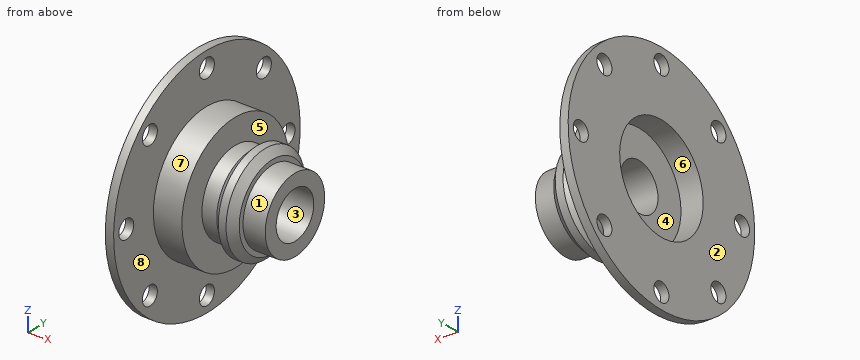
```python
from build123d import *

# Parameters (mm, degrees)
F2_R     = 4
F3_DEPTH = 3.551


with BuildPart() as f1:
    # F0 (on Front) → F1 (revolve)
    with BuildSketch(Plane.XZ):
        Polygon((-31.7, 10.0325), (0, 10.0325), (0, 15.85), (-9.5, 15.85), (-9.5, 17.875), (-12.625, 21), (-15.975, 21), (-19.1, 17.875), (-25.45, 17.875), (-25.45, 28.55), (-37.65, 28.55), (-37.65, 49.75), (-41.2, 49.75), (-41.2, 22.275), (-31.7, 22.275), align=None)
    revolve(axis=Axis((-20.6, 0, 0), (-1, 0, 0)))

    # F2 (on face) → F3 (cut, through all)
    with BuildSketch(Plane.YZ.offset(-37.65)):
        with Locations((0, 43)):
            Circle(F2_R)
        with Locations((30.405592, 30.405592)):
            Circle(F2_R)
        with Locations((43, 0)):
            Circle(F2_R)
        with Locations((30.405592, -30.405592)):
            Circle(F2_R)
        with Locations((0, -43)):
            Circle(F2_R)
        with Locations((-30.405592, -30.405592)):
            Circle(F2_R)
        with Locations((-43, 0)):
            Circle(F2_R)
        with Locations((-30.405592, 30.405592)):
            Circle(F2_R)
    extrude(amount=-F3_DEPTH, mode=Mode.SUBTRACT)


solid = f1.part
```
Geometry: final body of the model. Coordinates: model frame, mm. Face numbers are marked on the shaded views. A direction names the side the tool comes from. Coordinates: 2 decimals unless noted, no trailing zeros. Order: outer loops, then holes, each group sorted by start corner. A loop starts at its lowest first (then second) coordinate and runs counter-clockwise, first axis right, second up. Notation, with made-up numbers: (39.5, 40) -> (52.5, 40) arc R17 cw to (52.5, 55) -> close; hole circle Ø8 at (82.25, 64). An arc over 180 degrees is marked (long way). Answer in a Markdown table with one row per item.
Item 1: Contact query for flat-ended pins moving along their axis: P1, Ø9, axis at y = 0, z = -43, coming from the +X side; P2, Ø5, axis at x = -27, y = -3, coming from the +Z side; P3, Ø8, axis at x = -8.5, z = -9.5, coming from the +Y side. Output: stop coordinate, or through.
Return value:
| item | result |
|---|---|
| P1 | stops at x = -37.65 |
| P2 | stops at z = 28.55 |
| P3 | stops at y = 18.97 |
Item 2: Access query for the marked faces 1, 2, 3, 4 and 5. Directions: +Z, -Z, +X, -X, +Y, -Y. A direction counts if a zero-diameter tool reaches every point of the face in a straight line with its end or side. Return the directions, or none.
Return value:
| item | result |
|---|---|
| face 1 | +X |
| face 2 | +Z, -Z, -X, +Y, -Y |
| face 3 | +X, -X |
| face 4 | -X |
| face 5 | none |
Item 3: Ray query, L1, parallel to Y at x = -37.5, z = 0 (3 decimals); L2, parallel to X at y = 38, z = -17; L3, parallel to X at y = 10, z = -24.5. Return the intervals inside material, ascending.
Return value:
| item | result |
|---|---|
| L1 | y = -28.55 to -22.275, 22.275 to 28.55 |
| L2 | x = -41.2 to -37.65 |
| L3 | x = -41.2 to -25.45 |
Item 4: Section B-B on y = 31.5. Output: boundary loops of the cut face in (x, z).
Return value:
| item | result |
|---|---|
| outline | (-41.2, -38.51) -> (-37.65, -38.51) -> (-37.65, -34.25) -> (-41.2, -34.25) -> close; (-41.2, -26.56) -> (-37.65, -26.56) -> (-37.65, 26.56) -> (-41.2, 26.56) -> close; (-41.2, 34.25) -> (-37.65, 34.25) -> (-37.65, 38.51) -> (-41.2, 38.51) -> close |
Item 5: Section A-A on y = 43. Output: boundary loops of the cut face in (x, z), plus the area to 3 significant figures.
Return value:
| item | result |
|---|---|
| outline | (-41.2, -25.02) -> (-37.65, -25.02) -> (-37.65, -4) -> (-41.2, -4) -> close; (-41.2, 4) -> (-37.65, 4) -> (-37.65, 25.02) -> (-41.2, 25.02) -> close |
| area | 149 mm² |
Item 6: Section D-D on z = 0. State how many separate pieces and enclosed holes the cut face has, plus the area to 3 significant figures.
Return value:
| item | result |
|---|---|
| separate pieces | 4 |
| enclosed holes | 0 |
| area | 846 mm² |
Item 7: Draft query along Z for the marked faces 6, 7 and 8. Return one class per face: released by +Z, released by -Z, zero draft, split by the parting line, or undercut.
Return value:
| item | result |
|---|---|
| face 6 | undercut |
| face 7 | split by the parting line |
| face 8 | zero draft |
